```python
from build123d import *

# Parameters (mm, degrees)
SKETCH1_R           = 3.65
BOSS_EXTRUDE1_DEPTH = 500


with BuildPart() as part:
    # Sketch1 → Boss-Extrude1 (new body)
    with BuildSketch(Plane.XY):
        with BuildLine():
            Line((-15, -34), (-15, -43))
            ThreePointArc((-15, -43), (-14.414213562, -44.414213562), (-13, -45))
            Line((-13, -45), (-4, -45))
            Line((-4, -45), (-4, -42.5))
            Line((-4, -42.5), (-8.202216073, -42.5))
            Line((-8.202216073, -42.5), (-8.202216073, -39.955429293))
            Line((-8.202216073, -39.955429293), (-4.222649634, -35.975862854))
            Line((-4.222649634, -35.975862854), (4.222649634, -35.975862854))
            Line((4.222649634, -35.975862854), (8.202216073, -39.955429293))
            Line((8.202216073, -39.955429293), (8.202216073, -42.5))
            Line((8.202216073, -42.5), (4, -42.5))
            Line((4, -42.5), (4, -45))
            Line((4, -45), (13, -45))
            ThreePointArc((13, -45), (14.414213562, -44.414213562), (15, -43))
            Line((15, -43), (15, -34))
            Line((15, -34), (12.5, -34))
            Line((12.5, -34), (12.5, -38.202216073))
            Line((12.5, -38.202216073), (9.955429293, -38.202216073))
            Line((9.955429293, -38.202216073), (5.975862854, -34.222649634))
            Line((5.975862854, -34.222649634), (5.975862854, -25.777350366))
            Line((5.975862854, -25.777350366), (9.955429293, -21.797783927))
            Line((9.955429293, -21.797783927), (12.5, -21.797783927))
            Line((12.5, -21.797783927), (12.5, -26))
            Line((12.5, -26), (15, -26))
            Line((15, -26), (15, -4))
            Line((15, -4), (12.5, -4))
            Line((12.5, -4), (12.5, -8.202216073))
            Line((12.5, -8.202216073), (9.955429293, -8.202216073))
            Line((9.955429293, -8.202216073), (5.975862854, -4.222649634))
            Line((5.975862854, -4.222649634), (5.975862854, 4.222649634))
            Line((5.975862854, 4.222649634), (9.955429293, 8.202216073))
            Line((9.955429293, 8.202216073), (12.5, 8.202216073))
            Line((12.5, 8.202216073), (12.5, 4))
            Line((12.5, 4), (15, 4))
            Line((15, 4), (15, 13))
            ThreePointArc((15, 13), (14.414213562, 14.414213562), (13, 15))
            Line((13, 15), (4, 15))
            Line((4, 15), (4, 12.5))
            Line((4, 12.5), (8.202216073, 12.5))
            Line((8.202216073, 12.5), (8.202216073, 9.955429293))
            Line((8.202216073, 9.955429293), (4.222649634, 5.975862854))
            Line((4.222649634, 5.975862854), (-4.222649634, 5.975862854))
            Line((-4.222649634, 5.975862854), (-8.202216073, 9.955429293))
            Line((-8.202216073, 9.955429293), (-8.202216073, 12.5))
            Line((-8.202216073, 12.5), (-4, 12.5))
            Line((-4, 12.5), (-4, 15))
            Line((-4, 15), (-13, 15))
            ThreePointArc((-13, 15), (-14.414213562, 14.414213562), (-15, 13))
            Line((-15, 13), (-15, 4))
            Line((-15, 4), (-12.5, 4))
            Line((-12.5, 4), (-12.5, 8.202216073))
            Line((-12.5, 8.202216073), (-9.955429293, 8.202216073))
            Line((-9.955429293, 8.202216073), (-5.975862854, 4.222649634))
            Line((-5.975862854, 4.222649634), (-5.975862854, -4.222649634))
            Line((-5.975862854, -4.222649634), (-9.955429293, -8.202216073))
            Line((-9.955429293, -8.202216073), (-12.5, -8.202216073))
            Line((-12.5, -8.202216073), (-12.5, -4))
            Line((-12.5, -4), (-15, -4))
            Line((-15, -4), (-15, -26))
            Line((-15, -26), (-12.5, -26))
            Line((-12.5, -26), (-12.5, -21.797783927))
            Line((-12.5, -21.797783927), (-9.955429293, -21.797783927))
            Line((-9.955429293, -21.797783927), (-5.975862854, -25.777350366))
            Line((-5.975862854, -25.777350366), (-5.975862854, -34.222649634))
            Line((-5.975862854, -34.222649634), (-9.955429293, -38.202216073))
            Line((-9.955429293, -38.202216073), (-12.5, -38.202216073))
            Line((-12.5, -38.202216073), (-12.5, -34))
            Line((-12.5, -34), (-15, -34))
        make_face()
        with Locations((0, -30)):
            Circle(SKETCH1_R, mode=Mode.SUBTRACT)
        Circle(SKETCH1_R, mode=Mode.SUBTRACT)
        with BuildLine():
            Line((-10.463955813, -39.463955813), (-12.621642737, -39.463955813))
            ThreePointArc((-12.621642737, -39.463955813), (-13.328749519, -39.756849032), (-13.621642737, -40.463955813))
            Line((-13.621642737, -40.463955813), (-13.621642737, -42.621642737))
            ThreePointArc((-13.621642737, -42.621642737), (-13.328749519, -43.328749519), (-12.621642737, -43.621642737))
            Line((-12.621642737, -43.621642737), (-10.463955813, -43.621642737))
            ThreePointArc((-10.463955813, -43.621642737), (-9.756849032, -43.328749519), (-9.463955813, -42.621642737))
            Line((-9.463955813, -42.621642737), (-9.463955813, -40.463955813))
            ThreePointArc((-9.463955813, -40.463955813), (-9.756849032, -39.756849032), (-10.463955813, -39.463955813))
        make_face(mode=Mode.SUBTRACT)
        with BuildLine():
            Line((9.011119828, -9.620135349), (6.268756073, -6.877771595))
            ThreePointArc((6.268756073, -6.877771595), (5.944332724, -6.660998843), (5.561649292, -6.584878376))
            Line((5.561649292, -6.584878376), (-5.561649292, -6.584878376))
            ThreePointArc((-5.561649292, -6.584878376), (-5.944332724, -6.660998843), (-6.268756073, -6.877771595))
            Line((-6.268756073, -6.877771595), (-9.011119828, -9.620135349))
            ThreePointArc((-9.011119828, -9.620135349), (-9.335543176, -9.836908101), (-9.718226609, -9.913028568))
            Line((-9.718226609, -9.913028568), (-12.249589991, -9.913028568))
            ThreePointArc((-12.249589991, -9.913028568), (-12.956696772, -10.205921787), (-13.249589991, -10.913028568))
            Line((-13.249589991, -10.913028568), (-13.249589991, -19.086971432))
            ThreePointArc((-13.249589991, -19.086971432), (-12.956696772, -19.794078213), (-12.249589991, -20.086971432))
            Line((-12.249589991, -20.086971432), (-9.718226609, -20.086971432))
            ThreePointArc((-9.718226609, -20.086971432), (-9.335543176, -20.163091899), (-9.011119828, -20.379864651))
            Line((-9.011119828, -20.379864651), (-6.268756073, -23.122228405))
            ThreePointArc((-6.268756073, -23.122228405), (-5.944332724, -23.339001157), (-5.561649292, -23.415121624))
            Line((-5.561649292, -23.415121624), (5.561649292, -23.415121624))
            ThreePointArc((5.561649292, -23.415121624), (5.944332724, -23.339001157), (6.268756073, -23.122228405))
            Line((6.268756073, -23.122228405), (9.011119828, -20.379864651))
            ThreePointArc((9.011119828, -20.379864651), (9.335543176, -20.163091899), (9.718226609, -20.086971432))
            Line((9.718226609, -20.086971432), (12.249589991, -20.086971432))
            ThreePointArc((12.249589991, -20.086971432), (12.956696772, -19.794078213), (13.249589991, -19.086971432))
            Line((13.249589991, -19.086971432), (13.249589991, -10.913028568))
            ThreePointArc((13.249589991, -10.913028568), (12.956696772, -10.205921787), (12.249589991, -9.913028568))
            Line((12.249589991, -9.913028568), (9.718226609, -9.913028568))
            ThreePointArc((9.718226609, -9.913028568), (9.335543176, -9.836908101), (9.011119828, -9.620135349))
        make_face(mode=Mode.SUBTRACT)
        with BuildLine():
            Line((9.463955813, -40.463955813), (9.463955813, -42.621642737))
            ThreePointArc((9.463955813, -42.621642737), (9.756849032, -43.328749519), (10.463955813, -43.621642737))
            Line((10.463955813, -43.621642737), (12.621642737, -43.621642737))
            ThreePointArc((12.621642737, -43.621642737), (13.328749519, -43.328749519), (13.621642737, -42.621642737))
            Line((13.621642737, -42.621642737), (13.621642737, -40.463955813))
            ThreePointArc((13.621642737, -40.463955813), (13.328749519, -39.756849032), (12.621642737, -39.463955813))
            Line((12.621642737, -39.463955813), (10.463955813, -39.463955813))
            ThreePointArc((10.463955813, -39.463955813), (9.756849032, -39.756849032), (9.463955813, -40.463955813))
        make_face(mode=Mode.SUBTRACT)
        with BuildLine():
            Line((-9.463955813, 10.463955813), (-9.463955813, 12.621642737))
            ThreePointArc((-9.463955813, 12.621642737), (-9.756849032, 13.328749519), (-10.463955813, 13.621642737))
            Line((-10.463955813, 13.621642737), (-12.621642737, 13.621642737))
            ThreePointArc((-12.621642737, 13.621642737), (-13.328749519, 13.328749519), (-13.621642737, 12.621642737))
            Line((-13.621642737, 12.621642737), (-13.621642737, 10.463955813))
            ThreePointArc((-13.621642737, 10.463955813), (-13.328749519, 9.756849032), (-12.621642737, 9.463955813))
            Line((-12.621642737, 9.463955813), (-10.463955813, 9.463955813))
            ThreePointArc((-10.463955813, 9.463955813), (-9.756849032, 9.756849032), (-9.463955813, 10.463955813))
        make_face(mode=Mode.SUBTRACT)
        with BuildLine():
            Line((10.463955813, 9.463955813), (12.621642737, 9.463955813))
            ThreePointArc((12.621642737, 9.463955813), (13.328749519, 9.756849032), (13.621642737, 10.463955813))
            Line((13.621642737, 10.463955813), (13.621642737, 12.621642737))
            ThreePointArc((13.621642737, 12.621642737), (13.328749519, 13.328749519), (12.621642737, 13.621642737))
            Line((12.621642737, 13.621642737), (10.463955813, 13.621642737))
            ThreePointArc((10.463955813, 13.621642737), (9.756849032, 13.328749519), (9.463955813, 12.621642737))
            Line((9.463955813, 12.621642737), (9.463955813, 10.463955813))
            ThreePointArc((9.463955813, 10.463955813), (9.756849032, 9.756849032), (10.463955813, 9.463955813))
        make_face(mode=Mode.SUBTRACT)
    extrude(amount=BOSS_EXTRUDE1_DEPTH)


solid = part.part
```
Can you work these out from the model? Positions are in its coordinate system, mm. A direction names the side the tool comes from. Coordinates: 2 decimals unless noted, no trailing zeros.
1. I'm going to push flat-ended pins straight in: pin 1 (1.2 mm diameter, centred on x = -14, z = 263.5, fed in from +Y); pin 2 (2.5 mm diameter, centred on y = -32, z = 357.5, fed in from +X). Where does each tip first touch, or does it pass through?
2. Thinking about a two-plate mould opening in X: for faces 3 (the face through (0, -6.585, 246)), 4 (the face through (15, 8, 246)), 5 (the face through (-13.25, -15, 246)), 6 (the face through (-9, -45, 246)), which applies, +X half, -X half, draft (parallel to the pull), parting line (faces both ways), or undercut?
3. I need wall thicknesses on line 1 (X direction, y = -41, z = 319.5); line 2 (Y direction, x = 0, z = 294); line 3 (Y direction, x = -1.5, z = 258.5). Which ranges of each line are inside material? Lowest first, please.
4. If we section it at A-A (z = 110): Give the number of separate pieces and of enclosed holes in the cut face, then the cut area to 3 significant figures.
5. For faces 1 (the face through (0, -23.415, 246)), 2 (the face through (9, 15, 246)), which set-ups out of +Z, -Z, +X, -X, +Y, -Y let a thin tool reach every point of the face, with its end or its side?
Entries:
1. pin 1: stops at y = 14.96
1. pin 2: stops at x = 5.98
2. face 3: undercut
2. face 4: +X half
2. face 5: undercut
2. face 6: draft
3. line 1: x = -15 to -13.62, -9.46 to -8.2, 8.2 to 9.46, 13.62 to 15
3. line 2: y = -35.98 to -33.65, -26.35 to -23.42, -6.58 to -3.65, 3.65 to 5.98
3. line 3: y = -35.98 to -33.33, -26.67 to -23.42, -6.58 to -3.33, 3.33 to 5.98
4. separate pieces: 1
4. enclosed holes: 7
4. area: 610 mm2
5. face 1: +Z, -Z
5. face 2: +Z, -Z, +X, -X, +Y
